Here's how the part is built. I have some questions about the finished solid (model axes, mm). A direction names the side the tool comes from. Coordinates: 2 decimals unless noted, no trailing zeros. Loops run counter-clockwise (first coordinate to the right, second up) from the corner with the lowest first, then second, coordinate; pieces in that order, holes last.
```python
from build123d import *

# Parameters (mm, degrees)
CROQUIS2_R              = 50
SALIENTE_EXTRUIR1_DEPTH = 10
CROQUIS1_W              = 9.8
CROQUIS1_H              = 20.8
CROQUIS1_W_2            = 20.8
CROQUIS1_H_2            = 9.8
CORTAR_EXTRUIR3_DEPTH   = 72.414284285
CROQUIS4_R              = 7.75
CORTAR_EXTRUIR4_DEPTH   = 10
CROQUIS5_R              = 2.05
CORTAR_EXTRUIR5_DEPTH   = 10
CROQUIS6_R              = 2.05
CORTAR_EXTRUIR6_DEPTH   = 6


with BuildPart() as part:
    # Croquis2 → Saliente-Extruir1 (new body)
    with BuildSketch(Plane(origin=(0, 0, 0), x_dir=(0, 1, 0), z_dir=(0, 0, 1))):
        with Locations(Location((0, 0, 0), (0, 0, 270))):
            Circle(CROQUIS2_R)
    extrude(amount=SALIENTE_EXTRUIR1_DEPTH)

    # Croquis1 → Cortar-Extruir3 (cut, through all)
    with BuildSketch(Plane(origin=(0, 0, 0), x_dir=(0, 1, 0), z_dir=(0, 0, 1))):
        Polygon((15.964211374, 37.450825203), (5.564211374, 19.437496804), (14.051260331, 14.537496804), (24.451260331, 32.550825203), align=None)
        with Locations((0, 30)):
            Rectangle(CROQUIS1_W, CROQUIS1_H)
        Polygon((32.558561056, 24.464659221), (14.545232657, 14.064659221), (19.445232657, 5.577610264), (37.458561056, 15.977610264), align=None)
        with Locations((30.036606449, 0.021134743)):
            Rectangle(CROQUIS1_W_2, CROQUIS1_H_2)
        Polygon((37.487431651, -15.943076631), (19.474103253, -5.543076631), (14.574103253, -14.030125588), (32.587431651, -24.430125588), align=None)
        Polygon((24.50126567, -32.537426313), (14.10126567, -14.524097914), (5.614216713, -19.424097914), (16.014216713, -37.437426313), align=None)
        with Locations((0.057741191, -30.015471706)):
            Rectangle(CROQUIS1_W, CROQUIS1_H)
        Polygon((-15.906470183, -37.466296909), (-5.506470183, -19.45296851), (-13.99351914, -14.55296851), (-24.39351914, -32.566296909), align=None)
        Polygon((-32.500819864, -24.480130927), (-14.487491466, -14.080130927), (-19.387491466, -5.59308197), (-37.400819864, -15.99308197), align=None)
        with Locations((-29.978865257, -0.036606449)):
            Rectangle(CROQUIS1_W_2, CROQUIS1_H_2)
        Polygon((-37.42969046, 15.927604926), (-19.416362061, 5.527604926), (-14.516362061, 14.014653883), (-32.52969046, 24.414653883), align=None)
        Polygon((-24.443524479, 32.521954607), (-14.043524479, 14.508626209), (-5.556475521, 19.408626209), (-15.956475521, 37.421954607), align=None)
        with BuildLine():
            ThreePointArc((47.8, -1.200469891), (45.15, 1.449530109), (42.5, -1.200469891))
            ThreePointArc((42.5, -1.200469891), (40.916298266, -11.556282456), (36.848431426, -21.210474521))
            ThreePointArc((36.848431426, -21.210474521), (37.876754986, -24.76308434), (41.454989786, -23.827818822))
            ThreePointArc((41.454989786, -23.827818822), (46.039249889, -12.910019273), (47.8, -1.200469891))
        make_face()
        with BuildLine():
            ThreePointArc((1.200469891, 47.8), (-1.449530109, 45.15), (1.200469891, 42.5))
            ThreePointArc((1.200469891, 42.5), (11.556282456, 40.916298266), (21.210474521, 36.848431426))
            ThreePointArc((21.210474521, 36.848431426), (24.76308434, 37.876754986), (23.827818822, 41.454989786))
            ThreePointArc((23.827818822, 41.454989786), (12.910019273, 46.039249889), (1.200469891, 47.8))
        make_face()
        with BuildLine():
            ThreePointArc((-1.200469891, -47.8), (1.449530109, -45.15), (-1.200469891, -42.5))
            ThreePointArc((-1.200469891, -42.5), (-11.556282456, -40.916298266), (-21.210474521, -36.848431426))
            ThreePointArc((-21.210474521, -36.848431426), (-24.76308434, -37.876754986), (-23.827818822, -41.454989786))
            ThreePointArc((-23.827818822, -41.454989786), (-12.910019273, -46.039249889), (-1.200469891, -47.8))
        make_face()
        with BuildLine():
            ThreePointArc((-47.8, 1.200469891), (-45.15, -1.449530109), (-42.5, 1.200469891))
            ThreePointArc((-42.5, 1.200469891), (-40.916298266, 11.556282456), (-36.848431426, 21.210474521))
            ThreePointArc((-36.848431426, 21.210474521), (-37.876754986, 24.76308434), (-41.454989786, 23.827818822))
            ThreePointArc((-41.454989786, 23.827818822), (-46.039249889, 12.910019273), (-47.8, 1.200469891))
        make_face()
    extrude(amount=CORTAR_EXTRUIR3_DEPTH, mode=Mode.SUBTRACT)

    # Croquis4 → Cortar-Extruir4 (cut)
    with BuildSketch(Plane.XY.offset(10)):
        Circle(CROQUIS4_R)
    extrude(amount=-CORTAR_EXTRUIR4_DEPTH, mode=Mode.SUBTRACT)

    # Croquis5 → Cortar-Extruir5 (cut)
    with BuildSketch(Plane.XY.offset(10)):
        with Locations((0, 16)):
            Circle(CROQUIS5_R)
        with Locations((16, 0)):
            Circle(CROQUIS5_R)
        with Locations((0, -16)):
            Circle(CROQUIS5_R)
        with Locations((-16, 0)):
            Circle(CROQUIS5_R)
    extrude(amount=-CORTAR_EXTRUIR5_DEPTH, mode=Mode.SUBTRACT)

    # Croquis6 → Cortar-Extruir6 (cut)
    with BuildSketch(Plane.XY.offset(10)):
        with Locations((-32.17, 32.17)):
            Circle(CROQUIS6_R)
        with Locations((32.17, 32.17)):
            Circle(CROQUIS6_R)
        with Locations((32.17, -32.17)):
            Circle(CROQUIS6_R)
        with Locations((-32.17, -32.17)):
            Circle(CROQUIS6_R)
    extrude(amount=-CORTAR_EXTRUIR6_DEPTH, mode=Mode.SUBTRACT)


solid = part.part
```
1. We'd pull the mould along X, two halves only. Please class faces 1 (the flat face through (-1, -10, 0)), 2 (the flat face through (4.879, 30, 5)): +X half, -X half, draft (parallel to the pull), parting line (faces both ways), or undercut.
2. I want a section at A-A (y = -45.15). Please give me the cut outline in (x, z), then the cut area to 3 significant figures.
3. I want a section at C-C (z = 2.5). Give the number of separate pieces and of enclosed holes in the cut face, then the cut area to 3 significant figures.
4. For pin 1 (3.5 mm diameter, centred on x = 0, y = -16, fed in from +Z); pin 2 (2 mm diameter, centred on x = 13, z = 6, fed in from +Y); pin 3 (2 mm diameter, centred on x = 32.5, y = -33, fed in from +Z); pin 4 (3 mm diameter, centred on x = -32, z = 5, fed in from -Y), each with a flat end and sliding along its axis, tell me the tip position at first contact or that it passes through.
5. I want a section at B-B (x = -12). Please give me the cut outline in (y, z).
6. On a 3-axis mill with a long thin cutter (end or side, diameter ignored), from which of +Z, -Z, +X, -X, +Y, -Y can I reach the whole of each face in a straight line? I mean faces 3 (the cylindrical face through (-45.994, 13.07, 4.93)), 4 (the flat face through (-32, 32, 4)). Say none if no direction works.
7. I need wall thicknesses on line 1 along X through (y, z) = (9, 7.5); line 2 along Y through (x, z) = (-34, 2.5); line 3 along Y through (x, z) = (32.17, 7.1). Which ranges of each line are inside material? Lowest first, please.
Response values:
1. face 1: draft
1. face 2: undercut
2. outline: (-21.48, 0) - (-15.74, 0) - (-15.74, 10) - (-21.48, 10) - close; (1.45, 0) - (21.48, 0) - (21.48, 10) - (1.45, 10) - close
2. area: 258 mm2
3. separate pieces: 1
3. enclosed holes: 21
3. area: 4,610 mm2
4. pin 1: passes through
4. pin 2: stops at y = 48.54
4. pin 3: stops at z = 4
4. pin 4: stops at y = -39.62
5. outline: (-48.54, 0) - (-46.28, 0) - (-46.28, 10) - (-48.54, 10) - close; (-40.79, 0) - (-30.63, 0) - (-30.63, 10) - (-40.79, 10) - close; (-15.68, 0) - (15.74, 0) - (15.74, 10) - (-15.68, 10) - close; (30.57, 0) - (48.54, 0) - (48.54, 10) - (30.57, 10) - close
6. face 3: +Z, -Z
6. face 4: +Z
7. line 1: x = -49.18 to -46.96, -41.55 to -25.39, -17.45 to 17.47, 25.29 to 49.18
7. line 2: y = -36.66 to -21.88, -13.98 to -4.9, 4.9 to 13.97, 21.94 to 36.66
7. line 3: y = -38.28 to -34.22, -30.12 to -24.16, -12.85 to -4.84, 4.96 to 12.97, 24.29 to 30.12, 34.22 to 38.28
